Could you check a few things on this model? Use its own coordinates, in mm. A direction names the side the tool comes from. Round coordinates to 2 decimals unless told otherwise and drop trailing zeros. Write each loop counter-clockwise with the first axis right and the second up, starting at its lowest first coordinate (ties: lowest second). Pieces come first, ordered by that corner, then holes. Notation, with made-up numbers: (72, -3.75) - (115, -3.75) arc R19 cw to (115, 30.25) - close; hole circle Ø5 at (34.25, 83.25). An arc over 180 degrees is marked (long way). Write each question's results on one line, items separated by ' | '. Start each with the question number.
(1) On a 3-axis mill with a long thin cutter (end or side, diameter ignored), from which of +Z, -Z, +X, -X, +Y, -Y can I reach the whole of each face in a straight line? I mean faces 1 (the flat face through (0, 2, 2)), 2 (the flat face through (-2, 1, 0)). Say none if no direction works.
(2) Imagine slicing it at A-A on z = 0. Write out the boundary of the cut face in (x, y), then the cut area to 3 significant figures.
(3) Imagine slicing it at B-B on x = 0. Write out the boundary of the cut face in (y, z).
(4) Please list where these lines run through material, in increasing order: line 1 (X direction, y = 0.15, z = 0); line 2 (Z direction, x = -0.35, y = 0.7). Write a range as [from, to].
(5) For P1, Ø1, axis at x = -2, y = -1.5, coming from the +Z side; P2, Ø0.5, axis at x = -2.5, y = 1.5, coming from the -Z side; P3, Ø0.8, axis at x = 1.5, y = 1.5, coming from the -Z side, each with a flat end and sliding along its axis, tell me the tip position at first contact or that it passes through.
(6) Imagine slicing it at C-C on y = 0.15. Write out the boundary of the cut face in (x, z), then the cut area to 3 significant figures.
(7) Thinking about a two-plate mould opening in X: for faces 3 (the cylindrical face through (-1.2, 0.03, -0.05)), 4 (the conical face through (0.06, 1.88, 2.82)), 5 (the flat face through (-2, 1.5, 0.5)), which applies, +X half, -X half, draft (parallel to the pull), parting line (faces both ways), or undercut?
Autodesk Inventor part; units mm, degrees
ref_plane "YZ Plane" through (0, 0, 0) normal (1, 0, 0) x (0, 1, 0)
ref_plane "XZ Plane" through (0, 0, 0) normal (0, 1, 0) x (-1, 0, 0)
ref_plane "XY Plane" through (0, 0, 0) normal (0, 0, 1) x (1, 0, 0)
sketch "スケッチ1" plane through (0, 0, 0) normal (0, 0, 1) x (1, 0, 0)
  line L0 (1.2, -2) -> (1.2, 2)
  line L1 (1.2, 2) -> (2.7, 2)
  line L2 (2.7, 2) -> (3, 1.7)
  line L3 (3, 1.7) -> (3, -1.7)
  line L4 (0, 6.4765) -> (0, -6.4765) construction
  line L5 (3, -1.7) -> (2.7, -2)
  line L6 (2.7, -2) -> (1.2, -2)
  point P0 (0, 0)
  point P1 (0, 0)
  point P2 (0, 0)
  point P3 (1.2, 0)
  point P4 (3, 0)
  dimension "d0" = 6
  dimension "d1" = 2.4
  dimension "d2" = 4
  dimension "d3" = 0.3
  dimension "d4" = 0.3
revolve "回転1" add sketch "スケッチ1" angle 360 about axis through (0, 6.4765, 0) along (0, -1, 0)
sketch "スケッチ2" plane through (0, 2, 0) normal (0, 1, 0) x (1, 0, 0)
  line L0 (-3, -0.5) -> (3, -0.5)
  line L1 (3, -0.5) -> (3, 0.5)
  line L2 (3, 0.5) -> (-3, 0.5)
  line L3 (-3, 0.5) -> (-3, -0.5)
  line L4 (-3, -0.5) -> (3, 0.5) construction
  line L5 (3, -0.5) -> (-3, 0.5) construction
  circle A0 centre (0, 0) radius 3
  point P0 (0, 0)
  point P1 (2.958, -0.5)
  point P2 (2.958, 0.5)
  point P3 (-2.958, 0.5)
  point P4 (-2.958, -0.5)
  dimension "d6" = 1
extrude "押し出し1" cut sketch "スケッチ2" against normal blind 1 contours A0 L2 L0
equation "\"d4\" = d3"
properties part number "ARU-304S" material "ステンレス鋼 440C"
Response:
1) face 1: +Z, -Z, +X, -X, +Y | face 2: +X, -X, +Y
2) outline: (-3, -1.7) - (-2.7, -2) - (-1.2, -2) - (-1.2, 1) - (-3, 1) - close; (1.2, -2) - (2.7, -2) - (3, -1.7) - (3, 1) - (1.2, 1) - close | area: 10.7 mm²
3) outline: (-2, -2.7) - (-1.7, -3) - (1.7, -3) - (2, -2.7) - (2, -1.2) - (-2, -1.2) - close; (-2, 1.2) - (2, 1.2) - (2, 2.7) - (1.7, 3) - (-1.7, 3) - (-2, 2.7) - close
4) line 1: [-3, -1.2], [1.2, 3] | line 2: [-2.98, -1.15], [1.15, 2.98]
5) P1: z = 2.6 | P2: z = -1.98 | P3: z = -2.79
6) outline: circle Ø6 at (0, 0); hole circle Ø2.4 at (0, 0) | area: 23.8 mm²
7) face 3: undercut | face 4: parting line | face 5: draft
